Print and shaded views of the part. All mm, measured from the part's lowest x, y and z. A direction names the side the tool comes from. Give positions to 0.01 mm unless a question says otherwise; leave off trailing zeros. Order: outer loops, then holes, each group sorted by start corner. A loop starts at its lowest first (then second) coordinate and runs counter-clockwise, first axis right, second up. Notation, with made-up numbers: (41.5, 64) - (76.5, 64) arc R19 cw to (76.5, 68) - close; hole circle Ø6 at (-37.75, 21.5). An arc over 180 degrees is marked (long way). Answer in a Markdown table with one row per item.
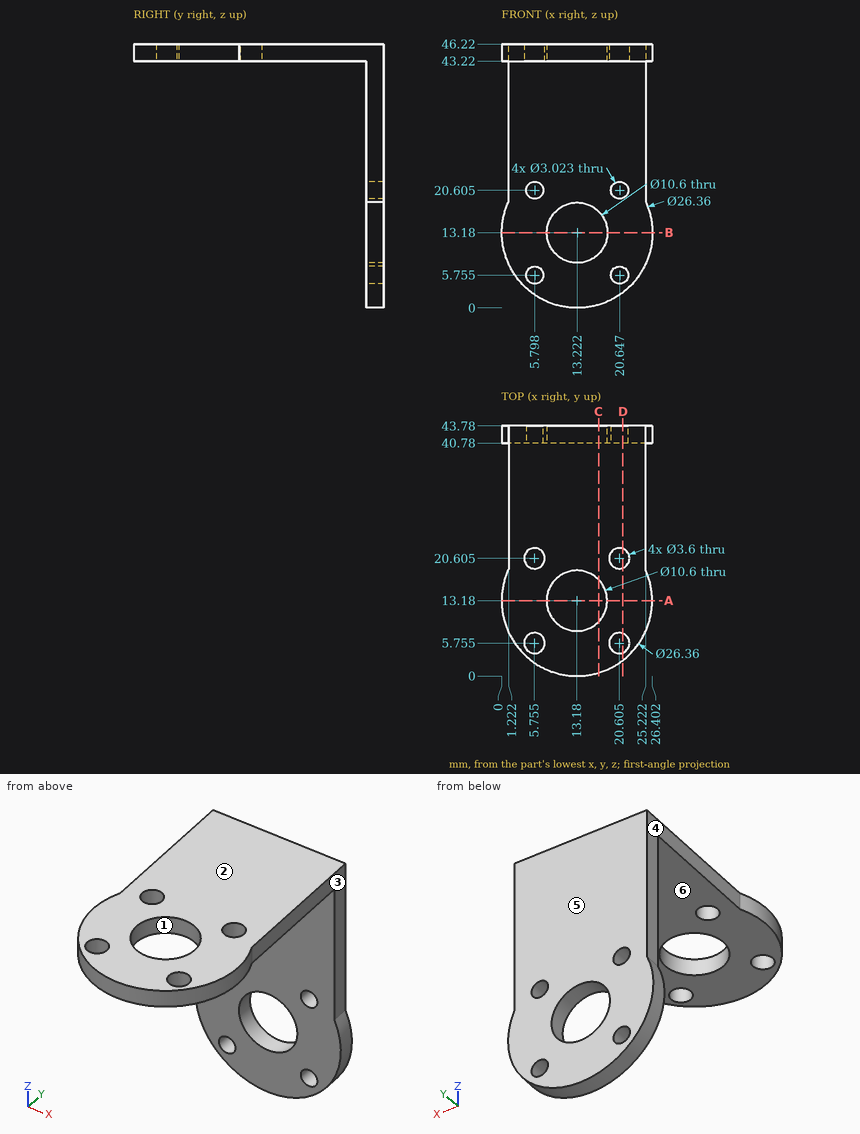
1. Cut at B-B on z = 13.18. Write the cut outline in (x, y).
Check result:
| item | result |
|---|---|
| outline | (0.04, 40.78) - (7.92, 40.78) - (7.92, 43.78) - (0.04, 43.78) - close; (18.52, 40.78) - (26.4, 40.78) - (26.4, 43.78) - (18.52, 43.78) - close |
2. Which spindle directions (+Z, -Z, +X, -X, +Y, -Y) get a long thin tool onto all of the face, cutting with end or side? Do the marked faces 5 and 6. Say none if no direction does.
Check result:
| item | result |
|---|---|
| face 5 | +Z, -Z, +X, -X, +Y |
| face 6 | -Z, +X, -X, -Y |
3. Cut at A-A on y = 13.18. Write the cut outline in (x, z).
Check result:
| item | result |
|---|---|
| outline | (0, 43.22) - (7.88, 43.22) - (7.88, 46.22) - (0, 46.22) - close; (18.48, 43.22) - (26.36, 43.22) - (26.36, 46.22) - (18.48, 46.22) - close |
4. Drop flat-ended pins along their axis: P1, Ø4, axis at x = 20.6, y = 5.76, coming from the -Z side; P2, Ø5, axis at x = 5.8, z = 20.6, coming from the +Y side; P3, Ø13, axis at x = 14, z = 24, coming from the -Y side. Give the stop position or say it passes through.
Check result:
| item | result |
|---|---|
| P1 | stops at z = 43.22 |
| P2 | stops at y = 43.78 |
| P3 | stops at y = 40.78 |
5. Cut at D-D on x = 21.25. Write the cut outline in (y, z) (1 decimal), and give its area (3 significant figures).
Check result:
| item | result |
|---|---|
| outline | (2.8, 43.2) - (4.1, 43.2) - (4.1, 46.2) - (2.8, 46.2) - close; (7.4, 43.2) - (18.9, 43.2) - (18.9, 46.2) - (7.4, 46.2) - close; (22.3, 43.2) - (40.8, 43.2) - (40.8, 22) - (43.8, 22) - (43.8, 46.2) - (22.3, 46.2) - close; (40.8, 2.7) - (43.8, 2.7) - (43.8, 4.4) - (40.8, 4.4) - close; (40.8, 7.1) - (43.8, 7.1) - (43.8, 19.2) - (40.8, 19.2) - close |
| area | 208 mm² |
6. Probe line 1 (X direction, y = 13.18, z = 45.1); line 2 (Y direction, x = 13.18, z = 45.35); line 3 (Y direction, x = 4, z = 41). List the from-to ranges inside material, lowest first.
Check result:
| item | result |
|---|---|
| line 1 | x = 0 to 7.88, 18.48 to 26.36 |
| line 2 | y = 0 to 7.88, 18.48 to 43.78 |
| line 3 | y = 40.78 to 43.78 |
7. Cut at C-C on x = 17. Write the cut outline in (y, z) (1 decimal).
Check result:
| item | result |
|---|---|
| outline | (0.6, 43.2) - (9.5, 43.2) - (9.5, 46.2) - (0.6, 46.2) - close; (16.9, 43.2) - (40.8, 43.2) - (40.8, 16.9) - (43.8, 16.9) - (43.8, 46.2) - (16.9, 46.2) - close; (40.8, 0.6) - (43.8, 0.6) - (43.8, 9.5) - (40.8, 9.5) - close |
8. Two-plate mould, pull along X, no slides. Class the marked faces 1, 2, 3 and 4: +X half, -X half, draft (parallel to the pull), parting line (faces both ways), or undercut.
Check result:
| item | result |
|---|---|
| face 1 | undercut |
| face 2 | draft |
| face 3 | +X half |
| face 4 | -X half |
